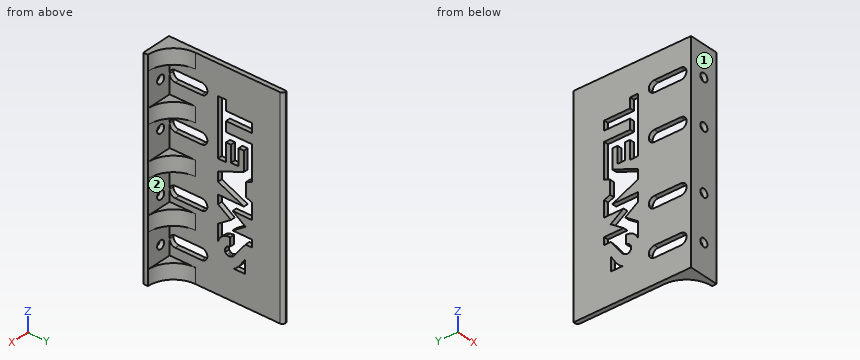
from build123d import *

# Parameters (mm, degrees)
SKETCH1_W           = 20
SKETCH1_H           = 140
BOSS_EXTRUDE1_DEPTH = 3
SKETCH2_W           = 3
SKETCH2_H           = 140
BOSS_EXTRUDE2_DEPTH = 75
SKETCH4_R           = 2.75
CUT_EXTRUDE1_DEPTH  = 10
CUT_EXTRUDE5_DEPTH  = 10
SKETCH13_W          = 7.5
SKETCH13_H          = 25
CUT_EXTRUDE6_DEPTH  = 162.161409773
BOSS_EXTRUDE3_DEPTH = 10
BOSS_EXTRUDE4_DEPTH = 5
FILLET1_R           = 3.75
BOSS_EXTRUDE5_DEPTH = 5
FILLET2_R           = 2


with BuildPart() as part:
    # Sketch1 → Boss-Extrude1 (new body)
    with BuildSketch(Plane(origin=(0, 0, 0), x_dir=(1, 0, 0), z_dir=(0, 1, 0))):
        with Locations((10, 70)):
            Rectangle(SKETCH1_W, SKETCH1_H)
    extrude(amount=BOSS_EXTRUDE1_DEPTH)

    # Sketch2 → Boss-Extrude2 (add)
    with BuildSketch(Plane(origin=(0, 3, 0), x_dir=(1, 0, 0), z_dir=(0, 1, 0))):
        with Locations((1.5, 70)):
            Rectangle(SKETCH2_W, SKETCH2_H)
    extrude(amount=BOSS_EXTRUDE2_DEPTH)

    # Sketch4 → Cut-Extrude1 (cut)
    with BuildSketch(Plane.XZ):
        with Locations(Location((10, -20, 0), (0, 0, 270))):
            Circle(SKETCH4_R)
        with Locations(Location((10, -50, 0), (0, 0, 270))):
            Circle(SKETCH4_R)
        with Locations(Location((10, -120, 0), (0, 0, 270))):
            Circle(SKETCH4_R)
        with Locations(Location((10, -90, 0), (0, 0, 270))):
            Circle(SKETCH4_R)
    extrude(amount=-CUT_EXTRUDE1_DEPTH, mode=Mode.SUBTRACT)

    # Sketch11 → Cut-Extrude5 (cut)
    with BuildSketch(Plane.ZY):
        Polygon((-19.87445306, 35.049470042), (-57.66845643, 35.049470042), (-57.66845643, 40.375700466), (-45.620710845, 40.375700466), (-45.620710845, 43.628558514), (-56.567955095, 43.628558514), (-56.567955095, 48.727655429), (-45.620710845, 48.727655429), (-45.620710845, 52.207646986), (-58.474335361, 52.207646986), (-65.4959872, 35.049470042), (-71.703981953, 35.049470042), (-79.431402399, 52.207646986), (-79.431402399, 35.049470042), (-85.289263166, 35.049470042), (-91.179988836, 43.628558514), (-97.088991148, 35.049470042), (-108.632759584, 35.049470042), (-106.964389123, 35.31022439), (-104.891781353, 36.405186985), (-103.26233135, 38.285640805), (-102.117236881, 40.724472664), (-101.911986572, 43.118576138), (-107.511545976, 43.118576138), (-108.014068376, 41.622730328), (-108.632759584, 40.724472664), (-109.956613224, 39.815464831), (-112.255625181, 39.815464831), (-113.41257384, 40.97241349), (-113.707994228, 41.740190554), (-113.707994228, 42.874973674), (-112.965179572, 44.700944573), (-112.077421007, 45.588703138), (-101.911986572, 53.280033045), (-101.911986572, 57.552931735), (-97.088991148, 57.552931735), (-97.088991148, 44.700944573), (-91.179988836, 53.280033045), (-85.289263166, 44.700944573), (-85.289263166, 57.552931735), (-74.691981497, 57.552931735), (-73.171666345, 53.601738278), (-64.027833458, 53.601738278), (-62.420466982, 57.552931735), (-39.437456147, 57.552931735), (-39.437456147, 40.375700466), (-32.711511222, 40.375700466), (-32.711511222, 57.552931735), (-26.571823468, 57.552931735), (-26.571823468, 40.375700466), (-19.87445306, 40.375700466), align=None)
        Polygon((-119.870983837, 52.978567636), (-111.030217867, 52.978567636), (-115.109674503, 50.296859936), (-115.872275446, 49.795549834), (-117.201338289, 48.727655429), (-119.05433748, 46.831756703), (-119.581300631, 46.026502002), (-119.870983837, 45.273325665), align=None)
    extrude(amount=-CUT_EXTRUDE5_DEPTH, mode=Mode.SUBTRACT)

    # Sketch13 → Cut-Extrude6 (cut, through all)
    with BuildSketch(Plane(origin=(3, 0, 0), x_dir=(0, 0, -1), z_dir=(1, 0, 0))):
        with Locations((20, 15.5)):
            Rectangle(SKETCH13_W, SKETCH13_H)
        with Locations((50, 15.5)):
            Rectangle(SKETCH13_W, SKETCH13_H)
        with Locations((90, 15.5)):
            Rectangle(SKETCH13_W, SKETCH13_H)
        with Locations((120, 15.5)):
            Rectangle(SKETCH13_W, SKETCH13_H)
    extrude(amount=-CUT_EXTRUDE6_DEPTH, mode=Mode.SUBTRACT)

    # Sketch14 → Boss-Extrude3 (add)
    with BuildSketch(Plane.XY):
        with BuildLine():
            Line((3, 3), (3, 20))
            ThreePointArc((3, 20), (7.97918472, 7.97918472), (20, 3))
            Line((20, 3), (3, 3))
        make_face()
    boss_extrude3 = extrude(amount=-BOSS_EXTRUDE3_DEPTH)

    # Mirror1: Boss-Extrude3 across plane
    add(boss_extrude3.mirror(Plane.XY.offset(-70)))

    # Sketch15 → Boss-Extrude4 (add, symmetric)
    with BuildSketch(Plane.XY.offset(-70)):
        with BuildLine():
            Line((3, 20), (3, 3))
            Line((3, 3), (20, 3))
            ThreePointArc((20, 3), (7.97918472, 7.97918472), (3, 20))
        make_face()
    extrude(amount=BOSS_EXTRUDE4_DEPTH, both=True)

    # Fillet1
    fillet1_edges = [part.edges().sort_by_distance(p)[0] for p in [
        (1.5, 3, -116.25),
        (1.5, 28, -116.25),
        (1.5, 28, -123.75),
        (1.5, 3, -123.75),
        (1.5, 3, -93.75),
        (1.5, 3, -86.25),
        (1.5, 28, -93.75),
        (1.5, 28, -86.25),
        (1.5, 3, -53.75),
        (1.5, 3, -46.25),
        (1.5, 28, -46.25),
        (1.5, 28, -53.75),
        (1.5, 3, -23.75),
        (1.5, 3, -16.25),
        (1.5, 28, -16.25),
        (1.5, 28, -23.75),
    ]]
    fillet(fillet1_edges, radius=FILLET1_R - 0.0001)  # a hair under: the kernel refuses the full size

    # Sketch16 → Boss-Extrude5 (add, symmetric)
    with BuildSketch(Plane(origin=(0, 0, -37.5), x_dir=(-1, 0, 0), z_dir=(0, 0, -1))):
        with BuildLine():
            Line((-20, 3), (-3, 3))
            Line((-3, 3), (-3, 20))
            ThreePointArc((-3, 20), (-7.97918472, 7.97918472), (-20, 3))
        make_face()
    boss_extrude5 = extrude(amount=BOSS_EXTRUDE5_DEPTH, both=True)

    # Mirror2: Boss-Extrude5 across plane
    add(boss_extrude5.mirror(Plane.XY.offset(-70)))

    # Fillet2
    fillet2_edges = [part.edges().sort_by_distance(p)[0] for p in [
        (3, 78, -70),
    ]]
    fillet(fillet2_edges, radius=FILLET2_R)


solid = part.part
Source: CAD feature listing. Evaluate the final solid. Frame: model axes, mm. Face numbers are marked on the shaded views. Give positions to 0.01 mm unless a question says otherwise; leave off trailing zeros. Write each loop counter-clockwise with the first axis right and the second up, starting at its lowest first coordinate (ties: lowest second). Pieces come first, ordered by that corner, then holes. Notation, with made-up numbers: M 37,39.25 L 92,39.25 A17 cw 92,44.25 Z; hole C -25.75,-35.5 d1. An arc over 180 degrees is marked long. Return JSON: item names as keys, results as strings. Group by question number.
1) Cut plane D-D, the plane x = 5.5. Output: boundary loops of the cut face in (y, z).
2) Cut plane C-C, the plane y = 18. Give the number of separate pieces and of enclosed holes in the cut face, then the cut area to 3 significant figures.
3) Cut plane A-A, the plane z = -83. Output: boundary loops of the cut face in (x, y), then the cut area to 3 significant figures.
4) Cut plane B-B, the plane x = 15. Output: boundary loops of the cut face in (y, z).
5) First-contact query: pin 1 Ø3.5 at (x, z) = (1, -98.5) entering from -Y; pin 2 Ø6 at (x, z) = (13, -62.5) entering from +Y; pin 3 Ø4 at (y, z) = (44.5, -54) entering from +X; pin 4 Ø12 at (x, z) = (13.5, -43.5) entering from +Y. Flat tips, straight axial feed; report the tip coordinate or a pass-through.
6) Ray query, L1, parallel to Z at x = 2, y = 17.5; L2, parallel to X at y = 1, z = -20; L3, parallel to X at y = 32.5, z = -106.5. Return the intervals inside material, ascending.
7) Draft query along Z for the marked faces 1 and 2. Return one class per face: released by +Z, released by -Z, zero draft, split by the parting line, or undercut.
Data:
{
 "1": {"outline": "M 0,-140 L 11.13,-140 L 11.13,-130 L 3,-130 L 3,-107.5 L 11.13,-107.5 L 11.13,-97.5 L 3,-97.5 L 3,-75 L 11.13,-75 L 11.13,-65 L 3,-65 L 3,-42.5 L 11.13,-42.5 L 11.13,-32.5 L 3,-32.5 L 3,-10 L 11.13,-10 L 11.13,0 L 0,0 Z"},
 "2": {"separate pieces": "5", "enclosed holes": "0", "area": "336 mm²"},
 "3": {"outline": "M 0,0 L 20,0 L 20,3 L 3,3 L 3,35.05 L 0,35.05 Z; M 0,57.55 L 3,57.55 L 3,76 A2 ccw 1,78 L 0,78 Z", "area": "217 mm²"},
 "4": {"outline": "M 0,-140 L 3.75,-140 L 3.75,-130 L 3,-130 L 3,-107.5 L 3.75,-107.5 L 3.75,-97.5 L 3,-97.5 L 3,-75 L 3.75,-75 L 3.75,-65 L 3,-65 L 3,-42.5 L 3.75,-42.5 L 3.75,-32.5 L 3,-32.5 L 3,-10 L 3.75,-10 L 3.75,0 L 0,0 Z"},
 "5": {"pin 1": "stops at y = 0", "pin 2": "stops at y = 5.37", "pin 3": "stops at x = 3", "pin 4": "stops at y = 8.39"},
 "6": {"L1": "z = -140 to -123.75, -116.25 to -93.75, -86.25 to -53.75, -46.25 to -23.75, -16.25 to 0", "L2": "x = 0 to 7.25, 12.75 to 20", "L3": "x = 0 to 3"},
 "7": {"face 1": "zero draft", "face 2": "undercut"}
}
